Can you work these out from the drawing? Everything is in mm from the part's minimum corner. A direction names the side the tool comes from. Coordinates: 2 decimals unless noted, no trailing zeros. Order: outer loops, then holes, each group sorted by start corner. A loop starts at its lowest first (then second) coordinate and runs counter-clockwise, first axis right, second up. Notation, with made-up numbers: (2.5, -35.75) -> (57.5, -35.75) arc R34 ccw to (57.5, -5.75) -> close; hole circle Ø1 at (-37, -4.5). An arc over 180 degrees is marked (long way). Write item = value, one per line. Start each with the question number.
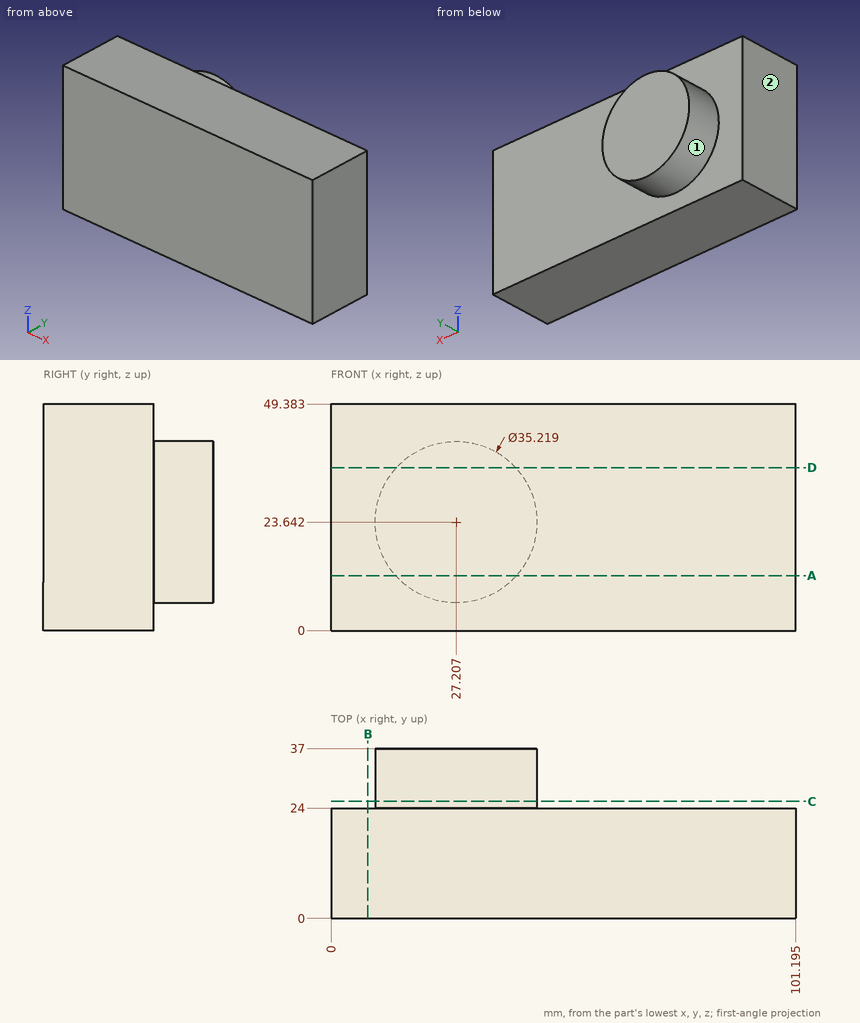
(1) For the marked faces 1 and 2, which set-ups out of +Z, -Z, +X, -X, +Y, -Y let a thin tool reach every point of the face, with its end or its side?
(2) Imagine slicing it at B-B (x = 8). Write out the boundary of the cut face in (y, z).
(3) If I drill on L1, parallel to Y at x = 53, z = 47; L2, parallel to X at y = 32, z = 17 (1 decimal); L3, parallel to X at y = 35, z = 14.5, over which ranges is the centre line in solid material (lowest first)? Write a range as from..to.
(4) Imagine slicing it at D-D (z = 35.5). Write out the boundary of the cut face in (x, y) (1 decimal).
(5) For P1, Ø8, axis at x = 20.5, y = 29, coming from the +Z side; P2, Ø1.5, axis at y = 28.5, z = 9.5, coming from the -X side, each with a flat end and sliding along its axis, tell me the tip position at first contact or that it passes through.
(6) Imagine slicing it at A-A (z = 12). Write out the boundary of the cut face in (x, y) (1 decimal), plus the area to 3 significant figures.
(7) Imagine slicing it at C-C (y = 25.5). Write out the boundary of the cut face in (x, z), plus the area to 3 significant figures.
Result set:
q1.face_1 = +Y
q1.face_2 = +Z, -Z, -X, +Y, -Y
q2.outline = (0, 0) -> (24, 0) -> (24, 49.38) -> (0, 49.38) -> close
q3.L1 = 0..24
q3.L2 = 10.9..43.5
q3.L3 = 12.16..42.26
q4.outline = (0, 0) -> (101.2, 0) -> (101.2, 24) -> (40.2, 24) -> (40.2, 37) -> (14.2, 37) -> (14.2, 24) -> (0, 24) -> close
q5.P1 = 41.04
q5.P2 = 15.77
q6.outline = (0, 0) -> (101.2, 0) -> (101.2, 24) -> (40.4, 24) -> (40.4, 37) -> (14, 37) -> (14, 24) -> (0, 24) -> close
q6.area = 2,770 mm2
q7.outline = circle Ø35.22 at (27.21, 23.64)
q7.area = 974 mm2
